Job drawing, mm, ordinate dimensions from the low corner. One solid piece. Coordinates: 2 decimals unless noted, no trailing zeros. Order: outer loops, then holes, each group sorted by start corner. A loop starts at its lowest first (then second) coordinate and runs counter-clockwise, first axis right, second up. Notation, with made-up numbers: (38, -17) - (79, -17) arc R29 cw to (79, 6) - close; hole circle Ø6 at (68, 16). An arc over 180 degrees is marked (long way). Use a Markdown table: item, result. Add a question column.
1) Saw through at A-A on y = 12.5. List the corners of the cut face in (x, z).
2) Saw through at C-C on z = 9. List the corners of the cut face in (x, y), then the cut area to 3 significant figures.
3) Saw through at D-D on y = 7.75. List the corners of the cut face in (x, z), then the cut area to 3 significant figures.
4) Saw through at B-B on x = 12.5. List the corners of the cut face in (y, z).
5) Two-plate mould, pull along X, no slides. Class the marked faces 1, 2 and 3: +X half, -X half, draft (parallel to the pull), parting line (faces both ways), or undercut.
6) Drop flat-ended pins along their axis: P1, Ø6, axis at x = 22.5, z = 29.5, coming from the -Y side; P2, Ø1.5, axis at x = 20, z = 30.5, coming from the -Y side; P3, Ø6.5, axis at x = 19.5, z = 9, coming from the +Y side; P4, Ø6.5, axis at x = 12.5, y = 12.5, coming from the -Z side. Give the stop position or say it passes through.
7) Wall check: L1, parallel to X at y = 9.75, z = 27.5; L2, parallel to X at y = 9.75, z = 8; L3, parallel to Y at x = 12.5, z = 15. Give the ranges that are in metal, low to high. Write a range as [from, to].
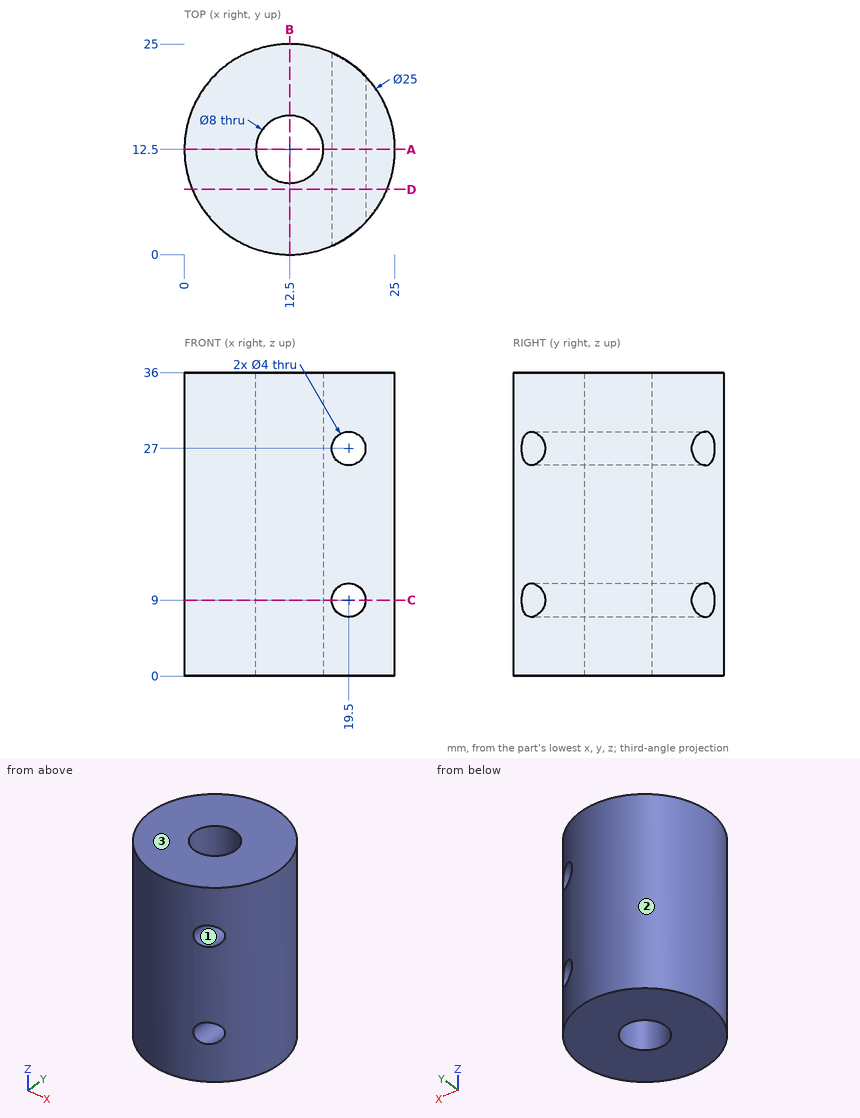
Results are:
| question | item | result |
|---|---|---|
| 1 | outline | (0, 0) - (8.5, 0) - (8.5, 36) - (0, 36) - close; (16.5, 0) - (25, 0) - (25, 36) - (16.5, 36) - close; hole circle Ø4 at (19.5, 9); hole circle Ø4 at (19.5, 27) |
| 2 | outline | (17.5, 1.04) - (17.5, 23.96) arc R12.5 ccw (long way) to start; (21.5, 3.83) arc R12.5 ccw to (21.5, 21.17) - close; hole circle Ø8 at (12.5, 12.5) |
| 2 | area | 359 mm2 |
| 3 | outline | (0.94, 0) - (24.06, 0) - (24.06, 36) - (0.94, 36) - close; hole circle Ø4 at (19.5, 9); hole circle Ø4 at (19.5, 27) |
| 3 | area | 807 mm2 |
| 4 | outline | (0, 0) - (8.5, 0) - (8.5, 36) - (0, 36) - close; (16.5, 0) - (25, 0) - (25, 36) - (16.5, 36) - close |
| 5 | face 1 | undercut |
| 5 | face 2 | parting line |
| 5 | face 3 | draft |
| 6 | P1 | y = 2.14 |
| 6 | P2 | y = 1.98 |
| 6 | P3 | y = 24.42 |
| 6 | P4 | through |
| 7 | L1 | [0.31, 9.6], [15.4, 17.56], [21.44, 24.69] |
| 7 | L2 | [0.31, 9.6], [15.4, 17.77], [21.23, 24.69] |
| 7 | L3 | [0, 8.5], [16.5, 25] |
